Part model, mm, in its own coordinate system. A direction names the side the tool comes from. Round coordinates to 2 decimals unless told otherwise and drop trailing zeros. Write each loop counter-clockwise with the first axis right and the second up, starting at its lowest first coordinate (ties: lowest second). Pieces come first, ordered by that corner, then holes. Notation, with made-up numbers: (12, 49.25) -> (60, 49.25) arc R21 cw to (60, 53.25) -> close; hole circle Ø5 at (15, 36). An arc over 180 degrees is marked (long way). Return JSON: item names as keys, results as strings. Group by question number.
(1) Drop flat-ended pins along their axis: pin 1 Ø6 at (x, y) = (3, 5) entering from -Z; pin 2 Ø3 at (y, z) = (6.5, -3) entering from -X; pin 3 Ø1.5 at (x, z) = (1.5, 1) entering from -Y; pin 4 Ø1.5 at (y, z) = (16, 4.5) entering from +X. Give the stop position or say it passes through.
(2) Tool access for faces 1 (the flat face through (2.3, 4, -2.5)), 2 (the flat face through (-2.535, 1.972, -4.31)): list every direction of +Z, -Z, +X, -X, +Y, -Y with a clear straight run to the whole face (end or side of a thin tool).
(3) Saw through at A-A (z = 0). List the corners of the cut face in (x, y).
(4) Drill centre lines: L1, parallel to Y at x = 0, z = 3.5; L2, parallel to Z at x = 0, y = 15.5; L3, parallel to X at y = 9, z = 1.5. Where is each one in solid material? Low to high. Write a range as from..to.
(5) Saw through at D-D (z = -4.5). List the corners of the cut face in (x, y), plus the area to 3 significant figures.
(6) Saw through at B-B (x = -1.5). List the corners of the cut face in (y, z).
(7) Saw through at C-C (y = 5.5). List the corners of the cut face in (x, z), plus the area to 3 significant figures.
Autodesk Inventor part; units mm, degrees
ref_plane "YZ Plane" through (0, 0, 0) normal (1, 0, 0) x (0, 1, 0)
ref_plane "XZ Plane" through (0, 0, 0) normal (0, 1, 0) x (-1, 0, 0)
ref_plane "XY Plane" through (0, 0, 0) normal (0, 0, 1) x (1, 0, 0)
sketch "Schizzo1" plane through (0, 0, 0) normal (0, 1, 0) x (-1, 0, 0)
  circle A0 centre (0, 0) radius 5
  line L0 (5, -2.8868) -> (0, -5.7735)
  line L1 (0, -5.7735) -> (-5, -2.8868)
  line L2 (-5, -2.8868) -> (-5, 2.8868)
  line L3 (-5, 2.8868) -> (0, 5.7735)
  line L4 (0, 5.7735) -> (5, 2.8868)
  line L5 (5, 2.8868) -> (5, -2.8868)
  point P0 (5, 0)
  dimension "d0" = 10
extrude "Estrusione1" add sketch "Schizzo1" along normal blind 4
sketch "Schizzo2" plane through (0, 4, 0) normal (0, 1, 0) x (1, 0, 0)
  circle A0 centre (0, 0) radius 3
  dimension "d3" = 6
extrude "Estrusione2" add sketch "Schizzo2" along normal blind 30
thread "Filettatura1"
properties part number "27_Vite_M6_30_Testa_Esagonale" material "Acciaio inox AISI 316"
Computed values:
{
 "1": {"pin 1": "z = -5.67", "pin 2": "x = -2.6", "pin 3": "y = 0", "pin 4": "through"},
 "2": {"face 1": "+Y", "face 2": "-Z, -X, +Y, -Y"},
 "3": {"outline": "(-5, 0) -> (5, 0) -> (5, 4) -> (3, 4) -> (3, 34) -> (-3, 34) -> (-3, 4) -> (-5, 4) -> close"},
 "4": {"L1": "0..4", "L2": "-3..3", "L3": "-2.6..2.6"},
 "5": {"outline": "(-2.21, 0) -> (2.21, 0) -> (2.21, 4) -> (-2.21, 4) -> close", "area": "17.6 mm2"},
 "6": {"outline": "(0, -4.91) -> (4, -4.91) -> (4, -2.6) -> (34, -2.6) -> (34, 2.6) -> (4, 2.6) -> (4, 4.91) -> (0, 4.91) -> close"},
 "7": {"outline": "circle Ø6 at (0, 0)", "area": "28.3 mm2"}
}
